Can you work these out from the model? Positions are in its coordinate system, mm. Face numbers are marked on the shaded views. Coordinates: 2 decimals unless noted, no trailing zeros. Write each loop counter-clockwise with the first axis right and the second up, starting at its lowest first coordinate (ties: lowest second). Pieces come first, ordered by that corner, then holes. Notation, with made-up numbers: M 84,59.25 L 138,59.25 A10 cw 138,66.25 Z; hole C 5.25,65.25 d8. An arc over 180 degrees is marked long. Answer as a JSON object with one key per item and string values. Group by question number.
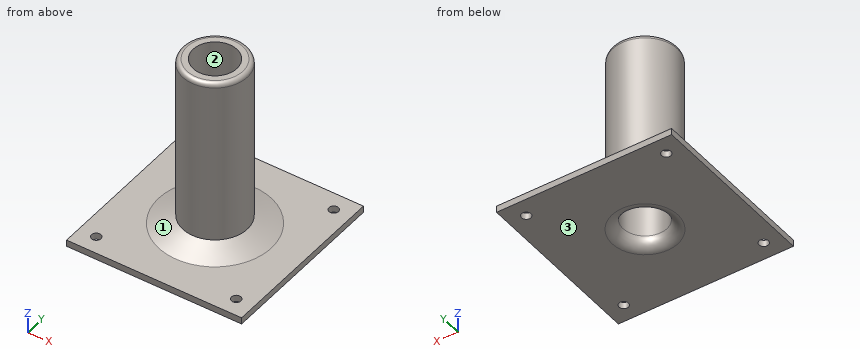
from build123d import *

# Parameters (mm, degrees)
ESQUISSE1_W                  = 80
ESQUISSE1_H                  = 80
BOSS_EXTRU_1_DEPTH           = 3
BOSS_EXTRU_2_START           = 3
ESQUISSE2_R                  = 14.75
BOSS_EXTRU_2_DEPTH           = 80
CONG_1_R                     = 2
CHANFREIN1_SIZE              = 4
CHANFREIN1_SIZE2             = 10.989909678
ENL_V_MAT_EXTRU_1_DEPTH      = 101.444014257
ENL_V_MAT_EXTRU_1_DEPTH_BACK = 101.444014257
ESQUISSE3_R                  = 10
CONG_2_R                     = 5
D_GAGEMENT_M43_D             = 4.3
SYM_TRIE2_COPY_1_D           = 4.3


with BuildPart() as part:
    # Esquisse1 → Boss.-Extru.1 (new body)
    with BuildSketch(Plane.XY):
        Rectangle(ESQUISSE1_W, ESQUISSE1_H)
    extrude(amount=BOSS_EXTRU_1_DEPTH)

    # Esquisse2 → Boss.-Extru.2 (add)
    with BuildSketch(Plane.XY.offset(BOSS_EXTRU_2_START)):
        with Locations(Location((0, 0, 0), (0, 0, 180))):
            Circle(ESQUISSE2_R)
    extrude(amount=BOSS_EXTRU_2_DEPTH)

    # Congé1
    cong_1_edges = [part.edges().sort_by_distance(p)[0] for p in [
        (14.75, 0, 83),
    ]]
    fillet(cong_1_edges, radius=CONG_1_R)

    # Chanfrein1
    chanfrein1_edges = [part.edges().sort_by_distance(p)[0] for p in [
        (14.75, 0, 3),
    ]]
    chanfrein1_side = [part.faces().sort_by_distance(p)[0] for p in [
        (14.75, 0, 42),
    ]]
    chamfer(chanfrein1_edges, length=CHANFREIN1_SIZE, length2=CHANFREIN1_SIZE2, reference=chanfrein1_side[0])

    # Esquisse3 → Enlèv. mat.-Extru.1 (cut, two sides: drawn at the far end of the back side and taken through both)
    with BuildSketch(Plane.XY.offset(-ENL_V_MAT_EXTRU_1_DEPTH_BACK)):
        with Locations(Location((0, 0, 0), (0, 0, 180))):
            Circle(ESQUISSE3_R)
    extrude(amount=ENL_V_MAT_EXTRU_1_DEPTH + ENL_V_MAT_EXTRU_1_DEPTH_BACK, mode=Mode.SUBTRACT)

    # Congé2
    cong_2_edges = [part.edges().sort_by_distance(p)[0] for p in [
        (10, 0, 0),
    ]]
    fillet(cong_2_edges, radius=CONG_2_R)

    # Dégagement M43 (through all)
    with Locations(Plane(origin=(3.971676253, 8.06271861, 3), x_dir=(1, 0, 0), z_dir=(0, 0, 1))):
        with Locations((28.028323747, -40.06271861)):
            d_gagement_m43 = Hole(D_GAGEMENT_M43_D / 2)

    # Symétrie1: Dégagement M43 across plane
    add(d_gagement_m43.mirror(Plane.ZX), mode=Mode.SUBTRACT)

    # Symétrie2: Dégagement M43 across plane
    add(d_gagement_m43.mirror(Plane(origin=(0, 0, 0), x_dir=(0, 0, 1), z_dir=(1, 0, 0))), mode=Mode.SUBTRACT)

    # Symétrie2 copy 1 (through all)
    with Locations(Plane(origin=(-3.971676253, -8.06271861, 3), x_dir=(-1, 0, 0), z_dir=(0, 0, 1))):
        with Locations((28.028323747, -40.06271861)):
            Hole(SYM_TRIE2_COPY_1_D / 2)


solid = part.part
Q1. If we section it at D-D on z = 68.5: List the corners of the cut face in (x, y) for me.
Q2. Will these pins go through, and if not, where does the flat tip stop? pin 1 (5 mm diameter, centred on x = -5, z = 60.5, fed in from +Y); pin 2 (5.5 mm diameter, centred on x = -32, y = 32, fed in from +Z); pin 3 (3 mm diameter, centred on y = -15, z = 29, fed in from -X).
Q3. We'd pull the mould along Y, two halves only. Please class the marked faces 1, 2 and 3: pulls with the +Y half, pulls with the -Y half, needs draft (parallel to the pull), parting line crosses it, or undercut.
Q4. If we section it at C-C on y = 0: List the corners of the cut face in (x, z) for me, and give its area (3 significant figures).
Q5. Please list where these lines run through material, in increasing order: L1, parallel to Y at x = 32, z = 1; L2, parallel to Y at x = 0, z = 35; L3, parallel to Y at x = 2.5, z = 41.
Q6. If we section it at A-A on y = 32: List the corners of the cut face in (x, z) for me, and give its area (3 significant figures).
Reply:
{
 "1": {"outline": "C 0,0 d29.5; hole C 0,0 d20"},
 "2": {"pin 1": "y = 14.54", "pin 2": "z = 3", "pin 3": "x = -5.94"},
 "3": {"face 1": "parting line crosses it", "face 2": "undercut", "face 3": "needs draft"},
 "4": {"outline": "M -40,0 L -15,0 A5 ccw -10,5 L -10,83 L -12.75,83 A2 ccw -14.75,81 L -14.75,7 L -25.74,3 L -40,3 Z; M 10,5 A5 ccw 15,0 L 40,0 L 40,3 L 25.74,3 L 14.75,7 L 14.75,81 A2 ccw 12.75,83 L 10,83 Z", "area": "972 mm^2"},
 "5": {"L1": "-40 to -34.15, -29.85 to 29.85, 34.15 to 40", "L2": "-14.75 to -10, 10 to 14.75", "L3": "-14.54 to -9.68, 9.68 to 14.54"},
 "6": {"outline": "M -40,0 L -34.15,0 L -34.15,3 L -40,3 Z; M -29.85,0 L 29.85,0 L 29.85,3 L -29.85,3 Z; M 34.15,0 L 40,0 L 40,3 L 34.15,3 Z", "area": "214 mm^2"}
}
